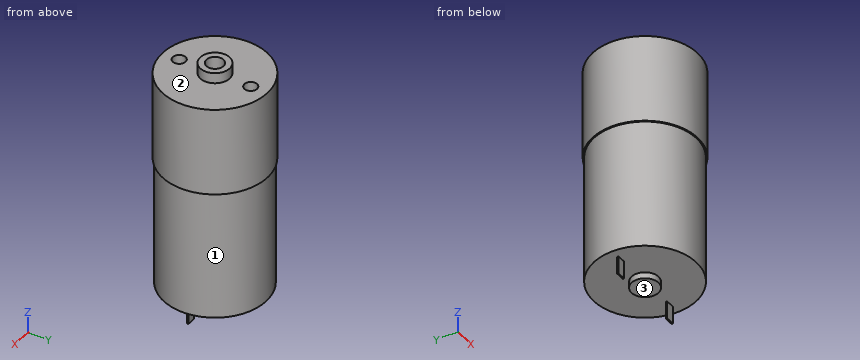
from build123d import *

# Parameters (mm, degrees)
F_01_START                                   = -21
S01_25_MM_47_TO_1_GEARBOX_R                  = 12.5
F_01_25_MM_47_TO_1_GEARBOX_DEPTH             = 21
F_02_START                                   = -51.8
S02_24_4_MM_MOTOR_CAN_R                      = 12.2
F_02_24_4_MM_MOTOR_CAN_DEPTH                 = 30.8
F_03_START                                   = -53.3
S03_REAR_SHAFT_BOSS_R                        = 3.2
F_03_REAR_SHAFT_BOSS_DEPTH                   = 1.5
F_04_START                                   = -56
S04_REAR_MOTOR_TERMINAL_1_W                  = 2.1
S04_REAR_MOTOR_TERMINAL_1_H                  = 0.3
F_04_REAR_MOTOR_TERMINAL_1_DEPTH             = 4.2
F_05_START                                   = -56
S05_REAR_MOTOR_TERMINAL_1_W                  = 2.1
S05_REAR_MOTOR_TERMINAL_1_H                  = 0.3
F_05_REAR_MOTOR_TERMINAL_1_DEPTH             = 4.2
F_06_START                                   = -6
S06_FACE_MOUNTING_M3_THREAD_ENVELOPES_R      = 1.52
F_06_FACE_MOUNTING_M3_THREAD_ENVELOPES_DEPTH = 6.1
S07_MOTOR_SHAFT_PILOT_R                      = 3.5
F_07_MOTOR_SHAFT_PILOT_DEPTH                 = 2.5
F_08_START                                   = -1
S08_OUTPUT_SHAFT_CLEARANCE_R                 = 2.03
F_08_OUTPUT_SHAFT_CLEARANCE_DEPTH            = 3.6


with BuildPart() as part:
    # S01 - 25 mm 47-to-1 gearbox → 01 - 25 mm 47-to-1 gearbox (new body)
    with BuildSketch(Plane.XY.offset(F_01_START)):
        with Locations(Location((0, 0, 0), (0, 0, 180))):
            Circle(S01_25_MM_47_TO_1_GEARBOX_R)
    extrude(amount=F_01_25_MM_47_TO_1_GEARBOX_DEPTH)

    # S02 - 24.4 mm motor can → 02 - 24.4 mm motor can (add)
    with BuildSketch(Plane.XY.offset(F_02_START)):
        with Locations(Location((0, 0, 0), (0, 0, 180))):
            Circle(S02_24_4_MM_MOTOR_CAN_R)
    extrude(amount=F_02_24_4_MM_MOTOR_CAN_DEPTH)

    # S03 - Rear shaft boss → 03 - Rear shaft boss (add)
    with BuildSketch(Plane.XY.offset(F_03_START)):
        Circle(S03_REAR_SHAFT_BOSS_R)
    extrude(amount=F_03_REAR_SHAFT_BOSS_DEPTH)

    # S04 - Rear motor terminal -1 → 04 - Rear motor terminal -1 (add)
    with BuildSketch(Plane.XY.offset(F_04_START)):
        with Locations((-9.05, 0)):
            Rectangle(S04_REAR_MOTOR_TERMINAL_1_W, S04_REAR_MOTOR_TERMINAL_1_H)
    extrude(amount=F_04_REAR_MOTOR_TERMINAL_1_DEPTH)

    # S05 - Rear motor terminal 1 → 05 - Rear motor terminal 1 (add)
    with BuildSketch(Plane.XY.offset(F_05_START)):
        with Locations((9.05, 0)):
            Rectangle(S05_REAR_MOTOR_TERMINAL_1_W, S05_REAR_MOTOR_TERMINAL_1_H)
    extrude(amount=F_05_REAR_MOTOR_TERMINAL_1_DEPTH)

    # S06 - Face mounting M3 thread envelopes → 06 - Face mounting M3 thread envelopes (cut)
    with BuildSketch(Plane.XY.offset(F_06_START)):
        with Locations((0, 8.5)):
            Circle(S06_FACE_MOUNTING_M3_THREAD_ENVELOPES_R)
        with Locations((0, -8.5)):
            Circle(S06_FACE_MOUNTING_M3_THREAD_ENVELOPES_R)
    extrude(amount=F_06_FACE_MOUNTING_M3_THREAD_ENVELOPES_DEPTH, mode=Mode.SUBTRACT)

    # S07 - Motor shaft pilot → 07 - Motor shaft pilot (add)
    with BuildSketch(Plane.XY):
        Circle(S07_MOTOR_SHAFT_PILOT_R)
    extrude(amount=F_07_MOTOR_SHAFT_PILOT_DEPTH)

    # S08 - Output shaft clearance → 08 - Output shaft clearance (cut)
    with BuildSketch(Plane.XY.offset(F_08_START)):
        Circle(S08_OUTPUT_SHAFT_CLEARANCE_R)
    extrude(amount=F_08_OUTPUT_SHAFT_CLEARANCE_DEPTH, mode=Mode.SUBTRACT)


solid = part.part
The listing builds one solid part. Answer for the finished solid, in the listing's coordinates (mm). Face numbers are marked on the shaded views. A direction names the side the tool comes from. Round coordinates to 2 decimals unless told otherwise and drop trailing zeros. Write each loop counter-clockwise with the first axis right and the second up, starting at its lowest first coordinate (ties: lowest second). Pieces come first, ordered by that corner, then holes. Notation, with made-up numbers: (-27, 87) - (25, 87) arc R10 cw to (25, 104) - close; hole circle Ø2 at (67.5, 0.25). An arc over 180 degrees is marked (long way). Use a Markdown table: item, result. Add a question column.
1. Consider line 1 (Y direction, x = 0, z = -3.8); line 2 (Y direction, x = 0, z = 0.6); line 3 (X direction, y = -0.5, z = -49). Determine where each line is inside the solid, lowest interval first.
2. Flat-ended cylindrical pins translate along their axes: P1, Ø2.5, axis at x = 9, z = -53.5, coming from the +Y side; P2, Ø6, axis at x = -2, y = 4, coming from the -Z side; P3, Ø5, axis at x = 1.5, z = -49.5, coming from the +Y side. Find the tip coordinate at first contact, or state that the pin passes through.
3. The part is cut by section B-B (y = -8.5). Write down the section's boundary in (x, z).
4. The part is cut by section A-A (x = 0). Write down the section's boundary in (y, z).
5. The part is cut by section D-D (x = -8.75). Write down the section's boundary in (y, z), and give its area (3 significant figures).
6. A tool of negligible diameter and unlimited length cuts with its end or side. For the marked faces 1, 2 and 3, from which of +Z, -Z, +X, -X, +Y, -Y can it reach the whole face along a straight path? Write none if from no direction.
7. The part is cut by section C-C (z = -45). Write down the section's boundary in (x, y), and give its area (3 significant figures).
Reported:
| question | item | result |
|---|---|---|
| 1 | line 1 | -12.5 to -10.02, -6.98 to 6.98, 10.02 to 12.5 |
| 1 | line 2 | -3.5 to -2.03, 2.03 to 3.5 |
| 1 | line 3 | -12.19 to 12.19 |
| 2 | P1 | y = 0.15 |
| 2 | P2 | z = -53.3 |
| 2 | P3 | y = 12.2 |
| 3 | outline | (-9.17, -21) - (-8.75, -21) - (-8.75, -51.8) - (8.75, -51.8) - (8.75, -21) - (9.17, -21) - (9.17, 0) - (1.52, 0) - (1.52, -6) - (-1.52, -6) - (-1.52, 0) - (-9.17, 0) - close |
| 4 | outline | (-12.5, -21) - (-12.2, -21) - (-12.2, -51.8) - (-3.2, -51.8) - (-3.2, -53.3) - (3.2, -53.3) - (3.2, -51.8) - (12.2, -51.8) - (12.2, -21) - (12.5, -21) - (12.5, 0) - (10.02, 0) - (10.02, -6) - (6.98, -6) - (6.98, 0) - (3.5, 0) - (3.5, 2.5) - (2.03, 2.5) - (2.03, -1) - (-2.03, -1) - (-2.03, 2.5) - (-3.5, 2.5) - (-3.5, 0) - (-6.98, 0) - (-6.98, -6) - (-10.02, -6) - (-10.02, 0) - (-12.5, 0) - close |
| 5 | outline | (-8.93, -21) - (-8.5, -21) - (-8.5, -51.8) - (-0.15, -51.8) - (-0.15, -56) - (0.15, -56) - (0.15, -51.8) - (8.5, -51.8) - (8.5, -21) - (8.93, -21) - (8.93, 0) - (-8.93, 0) - close |
| 5 | area | 900 mm^2 |
| 6 | face 1 | -Z |
| 6 | face 2 | +Z |
| 6 | face 3 | -Z, +Y, -Y |
| 7 | outline | circle Ø24.4 at (0, 0) |
| 7 | area | 468 mm^2 |
